from build123d import *

# Parameters (mm, degrees)
ESQUISSE1_W             = 130
ESQUISSE1_H             = 40
BASE_DEPTH              = 10
CHANFREIN1_SIZE         = 6
CHANFREIN2_SIZE         = 6
LANGUETTE_EXT_DEPTH     = 10
D_GAGEMENT_M31_D        = 30
ENL_V_MAT_EXTRU_1_REACH = 114.29
ESQUISSE5_W             = 20
ESQUISSE5_H             = 3
RAINURE_REACH           = 114.29
CONGES3MM_R             = 3
CONGES6MM_R             = 6


with BuildPart() as part:
    # Esquisse1 → Base (new body)
    with BuildSketch(Plane.XY):
        with Locations((13.160714286, 20)):
            Rectangle(ESQUISSE1_W, ESQUISSE1_H)
    extrude(amount=BASE_DEPTH)

    # Chanfrein1
    chanfrein1_edges = [part.edges().sort_by_distance(p)[0] for p in [
        (78.160714286, 0, 5),
    ]]
    chamfer(chanfrein1_edges, length=CHANFREIN1_SIZE)

    # Chanfrein2
    chanfrein2_edges = [part.edges().sort_by_distance(p)[0] for p in [
        (-51.839285714, 40, 5),
        (78.160714286, 40, 5),
        (-51.839285714, 0, 5),
    ]]
    chamfer(chanfrein2_edges, length=CHANFREIN2_SIZE)

    # languette → Languette_Ext (add)
    with BuildSketch(Plane(origin=(0, 0, 0), x_dir=(1, 0, 0), z_dir=(0, 1, 0))):
        with BuildLine():
            Line((-16.839285714, -10), (-16.839285714, 40))
            ThreePointArc((-16.839285714, 40), (13.160714286, 70), (43.160714286, 40))
            Line((43.160714286, 40), (43.160714286, -10))
            Line((43.160714286, -10), (-16.839285714, -10))
        make_face()
    extrude(amount=LANGUETTE_EXT_DEPTH)

    # Dégagement M31 (through all)
    with Locations(Plane(origin=(0, 0, 0), x_dir=(-1, 0, 0), z_dir=(0, -1, 0))):
        with Locations((-13.160714286, 40)):
            Hole(D_GAGEMENT_M31_D / 2)

    # Esquisse5 → Enlèv. mat.-Extru.1 (cut, up to next)
    with BuildSketch(Plane.XZ, mode=Mode.PRIVATE) as enl_v_mat_extru_1_sk1:
        with Locations((53.160714286, 8.5)):
            Rectangle(ESQUISSE5_W, ESQUISSE5_H)
    enl_v_mat_extru_1_tool1 = extrude(enl_v_mat_extru_1_sk1.sketch, amount=-ENL_V_MAT_EXTRU_1_REACH, mode=Mode.PRIVATE) & part.part
    enl_v_mat_extru_1 = enl_v_mat_extru_1_tool1.solids().sort_by_distance((53.160714, 0, 8.5))[0]
    add(enl_v_mat_extru_1, mode=Mode.SUBTRACT)

    # Symétrie1: Enlèv. mat.-Extru.1 across plane
    add(enl_v_mat_extru_1.mirror(Plane(origin=(13.160714286, 0, 0), x_dir=(0, 0, 1), z_dir=(1, 0, 0))), mode=Mode.SUBTRACT)

    # Esquisse7 → Rainure (cut, up to next)
    with BuildSketch(Plane(origin=(0, 0, 0), x_dir=(-1, 0, 0), z_dir=(0, 0, -1)), mode=Mode.PRIVATE) as rainure_sk1:
        with BuildLine():
            Line((-65.160714286, 28), (-51.160714286, 28))
            ThreePointArc((-51.160714286, 28), (-48.160714286, 25), (-51.160714286, 22))
            Line((-51.160714286, 22), (-65.160714286, 22))
            ThreePointArc((-65.160714286, 22), (-68.160714286, 25), (-65.160714286, 28))
        make_face()
    rainure_tool1 = extrude(rainure_sk1.sketch, amount=-RAINURE_REACH, mode=Mode.PRIVATE) & part.part
    rainure = rainure_tool1.solids().sort_by_distance((58.160714, 25, 0))[0]
    add(rainure, mode=Mode.SUBTRACT)

    # Symétrie2: Rainure across plane
    add(rainure.mirror(Plane(origin=(13.160714286, 0, 0), x_dir=(0, 0, 1), z_dir=(1, 0, 0))), mode=Mode.SUBTRACT)

    # Conges3mm
    conges3mm_edges = [part.edges().sort_by_distance(p)[0] for p in [
        (78.160714286, 20, 0),
        (75.160714286, 3, 0),
        (-51.839285714, 20, 0),
        (-31.339285714, 0, 0),
        (13.160714286, 40, 0),
        (75.160714286, 37, 0),
        (-48.839285714, 3, 0),
        (-48.839285714, 37, 0),
        (57.660714286, 0, 0),
        (13.160714286, 10, 0),
        (-16.839285714, 5, 0),
        (43.160714286, 5, 0),
        (43.160714286, 0, -20),
        (13.160714286, 0, -70),
        (-16.839285714, 0, -20),
        (43.160714286, 10, -20),
        (13.160714286, 10, -70),
        (-16.839285714, 10, -20),
    ]]
    fillet(conges3mm_edges, radius=CONGES3MM_R)

    # Conges6mm
    # the kernel refuses this fillet: 6 mm, written as the material it adds along each edge
    with BuildSketch(Plane(origin=(-36.839285714, 15.009618943, 7), x_dir=(1, 0, 0), z_dir=(0, 1, 0))) as conges6mm_piece_1_section:
        with BuildLine():
            CenterArc((5.196152423, -6), CONGES6MM_R, 90, 60)
            Line((0, -3), (0, 0))
            Line((0, 0), (5.196152423, 0))
        make_face()
    conges6mm_piece_1 = extrude(amount=37.980762114, mode=Mode.PRIVATE)
    conges6mm_piece_1 = split(conges6mm_piece_1, bisect_by=Plane(origin=(-34.649133292, 22, 7.793455272), z_dir=(0, -1, 0)), keep=Keep.TOP, mode=Mode.PRIVATE)
    add(conges6mm_piece_1)
    with BuildSketch(Plane(origin=(-36.839285714, 28, 7), x_dir=(1, 0, 0), z_dir=(0, 1, 0))) as conges6mm_piece_2:
        with BuildLine():
            CenterArc((5.196152423, -6), CONGES6MM_R, 90, 60)
            Line((0, -3), (0, 0))
            Line((0, 0), (5.196152423, 0))
        make_face()
    extrude(amount=12)
    with BuildSketch(Plane(origin=(-36.839285714, 0, 7), x_dir=(1, 0, 0), z_dir=(0, 1, 0))) as conges6mm_piece_3:
        with BuildLine():
            CenterArc((5.196152423, -6), CONGES6MM_R, 90, 60)
            Line((0, -3), (0, 0))
            Line((0, 0), (5.196152423, 0))
        make_face()
    extrude(amount=22)
    with BuildSketch(Plane(origin=(-36.839285714, -12.990381057, 7), x_dir=(1, 0, 0), z_dir=(0, 1, 0))) as conges6mm_piece_4_section:
        with BuildLine():
            CenterArc((5.196152423, -6), CONGES6MM_R, 90, 60)
            Line((0, -3), (0, 0))
            Line((0, 0), (5.196152423, 0))
        make_face()
    conges6mm_piece_4 = extrude(amount=47.980762114, mode=Mode.PRIVATE)
    conges6mm_piece_4 = split(conges6mm_piece_4, bisect_by=Plane(origin=(-34.649133292, 28, 7.793455272), z_dir=(0, 1, 0)), keep=Keep.TOP, mode=Mode.PRIVATE)
    add(conges6mm_piece_4)
    with BuildSketch(Plane(origin=(-16.839285714, 0, 7), x_dir=(0, 0, 1), z_dir=(0, 1, 0))) as conges6mm_piece_5_section:
        with BuildLine():
            CenterArc((6, -5.196152423), CONGES6MM_R, 120, 60)
            Line((0, -5.196152423), (0, 0))
            Line((0, 0), (3, 0))
        make_face()
    conges6mm_piece_5 = extrude(amount=40, mode=Mode.PRIVATE)
    conges6mm_piece_5 = conges6mm_piece_5 - Plane(origin=(-24.839285714, 25, 7.793455272), x_dir=(0, 1, 0), z_dir=(0, 0, -1)) * Cylinder(3, 101, mode=Mode.PRIVATE)
    add(conges6mm_piece_5)
    with BuildSketch(Plane(origin=(43.160714286, 0, 7), x_dir=(1, 0, 0), z_dir=(0, 1, 0))) as conges6mm_piece_6_section:
        with BuildLine():
            CenterArc((5.196152423, -6), CONGES6MM_R, 90, 60)
            Line((0, -3), (0, 0))
            Line((0, 0), (5.196152423, 0))
        make_face()
    conges6mm_piece_6 = extrude(amount=40, mode=Mode.PRIVATE)
    conges6mm_piece_6 = conges6mm_piece_6 - Plane(origin=(51.160714286, 25, 7.793455272), x_dir=(0, 1, 0), z_dir=(0, 0, -1)) * Cylinder(3, 101, mode=Mode.PRIVATE)
    add(conges6mm_piece_6)
    with BuildSketch(Plane(origin=(63.160714286, 0, 7), x_dir=(0, 0, 1), z_dir=(0, 1, 0))) as conges6mm_piece_7:
        with BuildLine():
            CenterArc((6, -5.196152423), CONGES6MM_R, 120, 60)
            Line((0, -5.196152423), (0, 0))
            Line((0, 0), (3, 0))
        make_face()
    extrude(amount=22)


solid = part.part
The model under review builds one solid part; all positions refer to its coordinate system, in mm. A direction names the side the tool comes from. Coordinates: 2 decimals unless noted, no trailing zeros. Write each loop counter-clockwise with the first axis right and the second up, starting at its lowest first coordinate (ties: lowest second). Pieces come first, ordered by that corner, then holes. Notation, with made-up numbers: (57.5, -7.5) - (87.5, -7.5) arc R24 ccw to (87.5, 18.5) - close; hole circle Ø9 at (81, 6). An arc over 180 degrees is marked (long way). Answer as a JSON object with one key per item and string values. Group by question number.
1. Add section C-C (x = 60.5). Give the boundary of the cut face in (y, z), plus the area to 3 significant figures.
2. Mouldability with a two-part tool opening along Y and no side actions: class faces 1 (the face through (68.16, 24.93, 4.93)), 2 (the face through (-48.28, 3.65, 0.9)), 3 (the face through (-51.839, 20, 6)) as pulls with the +Y half, pulls with the -Y half, needs draft (parallel to the pull), parting line crosses it, or undercut.
3. Clearance check with flat-ended pins moving along their axes: pin 1 Ø1 at (x, y) = (60.5, 33.5) entering from -Z; pin 2 Ø4.5 at (y, z) = (6, -17.5) entering from -X; pin 3 Ø10 at (x, z) = (18.5, -33) entering from +Y; pin 4 Ø10.5 at (x, y) = (51.5, 16) entering from +Z. State where each tip first meets the part, or that it passes through.
4. To check wall thickness, follow probe 1 along Z at (x, y) = (52, 34); probe 2 along Y at (x, z) = (0, -7). State the ranges of each line that lie inside material, in increasing order.
5. Machinability: for faces 4 (the face through (42.305, 9.098, -21.241)), 5 (the face through (61.003, 10.846, 7.826)), 6 (the face through (42.259, 0.855, -21.241)), which of the approach directions +Z, -Z, +X, -X, +Y, -Y give a long, thin tool a straight path to every point of the face, cutting with its end or side? Answer none if there is none.
6. Add section A-A (y = 14.5). Give the boundary of the cut face in (x, z), plus the area to 3 significant figures.
7. Add section B-B (z = -17). Give the boundary of the cut face in (x, y), plus the area to 3 significant figures.
Findings:
{
 "1": {"outline": "(0, 3) arc R3 ccw to (3, 0) - (22, 0) - (22, 7.56) - (0, 7.56) - close; (28, 0) - (37, 0) arc R3 ccw to (40, 3) - (40, 7) - (28, 7) - close", "area": "247 mm²"},
 "2": {"face 1": "undercut", "face 2": "pulls with the -Y half", "face 3": "needs draft"},
 "3": {"pin 1": "z = 0", "pin 2": "x = -16.84", "pin 3": "through", "pin 4": "z = 7.38"},
 "4": {"probe 1": "0 to 7", "probe 2": "0 to 10"},
 "5": {"face 4": "-Z, +X, +Y", "face 5": "+Z, +Y, -Y", "face 6": "-Z, +X, -Y"},
 "6": {"outline": "(-51.84, 3) arc R3 ccw to (-48.84, 0) - (75.16, 0) arc R3 ccw to (78.16, 3) - (78.16, 10) - (63.16, 10) arc R6 cw to (57.96, 7) - (48.36, 7) arc R6 cw to (43.16, 10) - (-16.84, 10) arc R6 cw to (-22.04, 7) - (-31.64, 7) arc R6 cw to (-36.84, 10) - (-51.84, 10) - close", "area": "1,190 mm²"},
 "7": {"outline": "(-16.84, 3) arc R3 ccw to (-13.84, 0) - (40.16, 0) arc R3 ccw to (43.16, 3) - (43.16, 7) arc R3 ccw to (40.16, 10) - (-13.84, 10) arc R3 ccw to (-16.84, 7) - close", "area": "592 mm²"}
}
